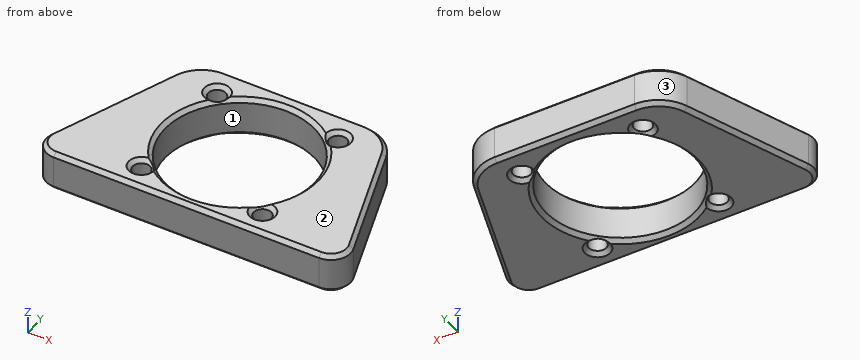
from build123d import *

# Parameters (mm, degrees)
SKETCH1_R           = 19
SKETCH1_R_2         = 2.25
BOSS_EXTRUDE1_DEPTH = 10
CHAMFER1_SIZE       = 1


with BuildPart() as part:
    # Sketch1 → Boss-Extrude1 (new body)
    with BuildSketch(Plane.XY):
        with BuildLine():
            Line((-27.380609914, 122.387194683), (-38.790304957, 90.693597341))
            ThreePointArc((-38.790304957, 90.693597341), (-38.176588293, 86.124933627), (-34.085867898, 84))
            Line((-34.085867898, 84), (-15.12911101, 84))
            Line((-15.12911101, 84), (15.12911101, 84))
            Line((15.12911101, 84), (34.085867898, 84))
            ThreePointArc((34.085867898, 84), (38.176588293, 86.124933627), (38.790304957, 90.693597341))
            Line((38.790304957, 90.693597341), (27.380609914, 122.387194683))
            ThreePointArc((27.380609914, 122.387194683), (23.721868541, 127.181440791), (17.971735796, 129))
            Line((17.971735796, 129), (-17.971735796, 129))
            ThreePointArc((-17.971735796, 129), (-23.721868541, 127.181440791), (-27.380609914, 122.387194683))
        make_face()
        with Locations(Location((0, 106, 0), (0, 0, 270))):
            Circle(SKETCH1_R, mode=Mode.SUBTRACT)
        with Locations(Location((15.556349182, 90.443650818, 0), (0, 0, 270))):
            Circle(SKETCH1_R_2, mode=Mode.SUBTRACT)
        with Locations(Location((-15.556349182, 90.443650818, 0), (0, 0, 270))):
            Circle(SKETCH1_R_2, mode=Mode.SUBTRACT)
        with Locations(Location((15.556349182, 121.556349182, 0), (0, 0, 270))):
            Circle(SKETCH1_R_2, mode=Mode.SUBTRACT)
        with Locations(Location((-15.556349182, 121.556349182, 0), (0, 0, 270))):
            Circle(SKETCH1_R_2, mode=Mode.SUBTRACT)
    extrude(amount=BOSS_EXTRUDE1_DEPTH)

    # Chamfer1
    # the kernel refuses this chamfer: 1 mm, written as the material it takes off along each edge
    with BuildSketch(Plane(origin=(17.971735796, 129, 0), x_dir=(0, 0.027495876610582174, 0.9996219169112968), z_dir=(-1, 0, 0)), Plane(origin=(17.971735796, 129, 10), x_dir=(0, -0.9996219169112968, 0.02749587661058574), z_dir=(-1, 0, 0))) as chamfer1_piece_1:
        Polygon((CHAMFER1_SIZE * 0.999621916911, -CHAMFER1_SIZE * 0.0274958766106), (-CHAMFER1_SIZE * 0.0274958766106, -CHAMFER1_SIZE * 0.999621916911), (0, 0), align=None)
    extrude(amount=35.943471591, mode=Mode.SUBTRACT)
    with BuildSketch(Plane(origin=(17.971735796, 119, 0), x_dir=(0.9408874118687268, 0.33871946827274174, 0), z_dir=(0.33871946827274174, -0.9408874118687268, 0))) as chamfer1_piece_2:
        Polygon((10, CHAMFER1_SIZE), (10 - CHAMFER1_SIZE, 0), (10, 0), align=None)
    revolve(axis=Axis((17.971735796, 119, 0), (0, 0, 1)), revolution_arc=70.201123645, mode=Mode.SUBTRACT)
    with BuildSketch(Plane(origin=(38.790304957, 90.693597341, 0), x_dir=(0.025870524181196484, 0.009313388705230746, 0.9996219169112968), z_dir=(-0.3387194682727421, 0.9408874118687267, 0)), Plane(origin=(-27.380609914, 122.387194683, 0), x_dir=(-0.025870524181196484, 0.00931338870523073, 0.9996219169112968), z_dir=(-0.3387194682727416, -0.9408874118687268, 0)), Plane(origin=(38.790304957, 90.693597341, 10), x_dir=(-0.9405316782499255, -0.33859140416997363, 0.027495876610585557), z_dir=(-0.3387194682727421, 0.9408874118687267, 0))) as chamfer1_piece_3:
        Polygon((CHAMFER1_SIZE * 0.999621916911, -CHAMFER1_SIZE * 0.0274958766106), (-CHAMFER1_SIZE * 0.0274958766106, -CHAMFER1_SIZE * 0.999621916911), (0, 0), align=None)
    extrude(amount=33.684792613, mode=Mode.SUBTRACT)
    with BuildSketch(Plane(origin=(34.085867898, 89, 0), x_dir=(0, -1, 0), z_dir=(-1, 0, 0))) as chamfer1_piece_4:
        Polygon((5, CHAMFER1_SIZE), (5 - CHAMFER1_SIZE, 0), (5, 0), align=None)
    revolve(axis=Axis((34.085867898, 89, 0), (0, 0, 1)), revolution_arc=109.798876355, mode=Mode.SUBTRACT)
    with BuildSketch(Plane(origin=(-34.085867898, 84, 0), x_dir=(0, -0.027495876610582174, 0.9996219169112968), z_dir=(1, 0, 0))) as chamfer1_piece_5:
        Polygon((CHAMFER1_SIZE * 0.999621916911, -CHAMFER1_SIZE * 0.0274958766106), (-CHAMFER1_SIZE * 0.0274958766106, -CHAMFER1_SIZE * 0.999621916911), (0, 0), align=None)
    extrude(amount=68.171735796, mode=Mode.SUBTRACT)
    with BuildSketch(Plane(origin=(-34.085867898, 89, 0), x_dir=(-0.9408874118687287, 0.33871946827273663, 0), z_dir=(0.33871946827273663, 0.9408874118687287, 0))) as chamfer1_piece_6:
        Polygon((5 - CHAMFER1_SIZE, 0), (5, CHAMFER1_SIZE), (5, 0), align=None)
    revolve(axis=Axis((-34.085867898, 89, 0), (0, 0, 1)), revolution_arc=109.798876355, mode=Mode.SUBTRACT)
    with BuildSketch(Plane(origin=(-17.971735796, 119, 0), x_dir=(0, 1, 0), z_dir=(1, 0, 0))) as chamfer1_piece_7:
        Polygon((10 - CHAMFER1_SIZE, 0), (10, CHAMFER1_SIZE), (10, 0), align=None)
    revolve(axis=Axis((-17.971735796, 119, 0), (0, 0, 1)), revolution_arc=70.201123645, mode=Mode.SUBTRACT)
    with BuildSketch(Plane(origin=(0, 106, 0), x_dir=(0, -1, 0), z_dir=(-1, 0, 0))) as chamfer1_piece_8:
        Polygon((19, CHAMFER1_SIZE), (19 + CHAMFER1_SIZE, 0), (19, 0), align=None)
    revolve(axis=Axis((0, 106, 0), (0, 0, 1)), mode=Mode.SUBTRACT)
    with BuildSketch(Plane(origin=(15.556349182, 90.443650818, 0), x_dir=(0, -1, 0), z_dir=(-1, 0, 0))) as chamfer1_piece_9:
        Polygon((2.25, CHAMFER1_SIZE), (2.25 + CHAMFER1_SIZE, 0), (2.25, 0), align=None)
    revolve(axis=Axis((15.556349182, 90.443650818, 0), (0, 0, 1)), mode=Mode.SUBTRACT)
    with BuildSketch(Plane(origin=(-15.556349182, 90.443650818, 0), x_dir=(0, -1, 0), z_dir=(-1, 0, 0))) as chamfer1_piece_10:
        Polygon((2.25, CHAMFER1_SIZE), (2.25 + CHAMFER1_SIZE, 0), (2.25, 0), align=None)
    revolve(axis=Axis((-15.556349182, 90.443650818, 0), (0, 0, 1)), mode=Mode.SUBTRACT)
    with BuildSketch(Plane(origin=(15.556349182, 121.556349182, 0), x_dir=(0, -1, 0), z_dir=(-1, 0, 0))) as chamfer1_piece_11:
        Polygon((2.25, CHAMFER1_SIZE), (2.25 + CHAMFER1_SIZE, 0), (2.25, 0), align=None)
    revolve(axis=Axis((15.556349182, 121.556349182, 0), (0, 0, 1)), mode=Mode.SUBTRACT)
    with BuildSketch(Plane(origin=(-15.556349182, 121.556349182, 0), x_dir=(0, -1, 0), z_dir=(-1, 0, 0))) as chamfer1_piece_12:
        Polygon((2.25, CHAMFER1_SIZE), (2.25 + CHAMFER1_SIZE, 0), (2.25, 0), align=None)
    revolve(axis=Axis((-15.556349182, 121.556349182, 0), (0, 0, 1)), mode=Mode.SUBTRACT)
    with BuildSketch(Plane(origin=(-17.971735796, 119, 10), x_dir=(0, 1, 0), z_dir=(1, 0, 0))) as chamfer1_piece_13:
        Polygon((10 - CHAMFER1_SIZE, 0), (10, -CHAMFER1_SIZE), (10, 0), align=None)
    revolve(axis=Axis((-17.971735796, 119, 10), (0, 0, 1)), revolution_arc=70.201123645, mode=Mode.SUBTRACT)
    with BuildSketch(Plane(origin=(-27.380609914, 122.387194683, 10), x_dir=(-0.025870524181196505, 0.009313388705230739, -0.9996219169112968), z_dir=(-0.3387194682727416, -0.9408874118687268, 0))) as chamfer1_piece_14:
        Polygon((CHAMFER1_SIZE * 0.999621916911, CHAMFER1_SIZE * 0.0274958766106), (-CHAMFER1_SIZE * 0.0274958766106, CHAMFER1_SIZE * 0.999621916911), (0, 0), align=None)
    extrude(amount=33.684792613, mode=Mode.SUBTRACT)
    with BuildSketch(Plane(origin=(-34.085867898, 89, 10), x_dir=(-0.9408874118687287, 0.33871946827273663, 0), z_dir=(0.33871946827273663, 0.9408874118687287, 0))) as chamfer1_piece_15:
        Polygon((5 - CHAMFER1_SIZE, 0), (5, -CHAMFER1_SIZE), (5, 0), align=None)
    revolve(axis=Axis((-34.085867898, 89, 10), (0, 0, 1)), revolution_arc=109.798876355, mode=Mode.SUBTRACT)
    with BuildSketch(Plane(origin=(34.085867898, 84, 10), x_dir=(0, 0.9996219169112968, 0.02749587661058574), z_dir=(-1, 0, 0))) as chamfer1_piece_16:
        Polygon((CHAMFER1_SIZE * 0.999621916911, CHAMFER1_SIZE * 0.0274958766106), (-CHAMFER1_SIZE * 0.0274958766106, CHAMFER1_SIZE * 0.999621916911), (0, 0), align=None)
    extrude(amount=68.171735796, mode=Mode.SUBTRACT)
    with BuildSketch(Plane(origin=(34.085867898, 89, 10), x_dir=(0, -1, 0), z_dir=(-1, 0, 0))) as chamfer1_piece_17:
        Polygon((5 - CHAMFER1_SIZE, 0), (5, -CHAMFER1_SIZE), (5, 0), align=None)
    revolve(axis=Axis((34.085867898, 89, 10), (0, 0, 1)), revolution_arc=109.798876355, mode=Mode.SUBTRACT)
    with BuildSketch(Plane(origin=(17.971735796, 119, 10), x_dir=(0.9408874118687268, 0.33871946827274174, 0), z_dir=(0.33871946827274174, -0.9408874118687268, 0))) as chamfer1_piece_18:
        Polygon((10 - CHAMFER1_SIZE, 0), (10, -CHAMFER1_SIZE), (10, 0), align=None)
    revolve(axis=Axis((17.971735796, 119, 10), (0, 0, 1)), revolution_arc=70.201123645, mode=Mode.SUBTRACT)
    with BuildSketch(Plane(origin=(0, 106, 10), x_dir=(0, -1, 0), z_dir=(-1, 0, 0))) as chamfer1_piece_19:
        Polygon((19 + CHAMFER1_SIZE, 0), (19, -CHAMFER1_SIZE), (19, 0), align=None)
    revolve(axis=Axis((0, 106, 10), (0, 0, 1)), mode=Mode.SUBTRACT)
    with BuildSketch(Plane(origin=(15.556349182, 90.443650818, 10), x_dir=(0, -1, 0), z_dir=(-1, 0, 0))) as chamfer1_piece_20:
        Polygon((2.25 + CHAMFER1_SIZE, 0), (2.25, -CHAMFER1_SIZE), (2.25, 0), align=None)
    revolve(axis=Axis((15.556349182, 90.443650818, 10), (0, 0, 1)), mode=Mode.SUBTRACT)
    with BuildSketch(Plane(origin=(-15.556349182, 90.443650818, 10), x_dir=(0, -1, 0), z_dir=(-1, 0, 0))) as chamfer1_piece_21:
        Polygon((2.25 + CHAMFER1_SIZE, 0), (2.25, -CHAMFER1_SIZE), (2.25, 0), align=None)
    revolve(axis=Axis((-15.556349182, 90.443650818, 10), (0, 0, 1)), mode=Mode.SUBTRACT)
    with BuildSketch(Plane(origin=(15.556349182, 121.556349182, 10), x_dir=(0, -1, 0), z_dir=(-1, 0, 0))) as chamfer1_piece_22:
        Polygon((2.25 + CHAMFER1_SIZE, 0), (2.25, -CHAMFER1_SIZE), (2.25, 0), align=None)
    revolve(axis=Axis((15.556349182, 121.556349182, 10), (0, 0, 1)), mode=Mode.SUBTRACT)
    with BuildSketch(Plane(origin=(-15.556349182, 121.556349182, 10), x_dir=(0, -1, 0), z_dir=(-1, 0, 0))) as chamfer1_piece_23:
        Polygon((2.25 + CHAMFER1_SIZE, 0), (2.25, -CHAMFER1_SIZE), (2.25, 0), align=None)
    revolve(axis=Axis((-15.556349182, 121.556349182, 10), (0, 0, 1)), mode=Mode.SUBTRACT)


solid = part.part
Check sheet for the modelled part. Datum: model origin and axes. Units: mm. Face numbers are marked on the shaded views. Give positions to 0.01 mm unless a question says otherwise; leave off trailing zeros. Write each loop counter-clockwise with the first axis right and the second up, starting at its lowest first coordinate (ties: lowest second). Pieces come first, ordered by that corner, then holes. Notation, with made-up numbers: (41, 21) -> (78, 21) arc R34 cw to (78, 54) -> close; hole circle Ø5 at (26.25, -22). An arc over 180 degrees is marked (long way). Write item = value, one per line.
Item 1: Sectioned sample at C-C on y = 106. Record the boundary of the cut face in (x, z).
Output:
outline = (-33.28, 1) -> (-32.22, 0) -> (-20, 0) -> (-19, 1) -> (-19, 9) -> (-20, 10) -> (-32.22, 10) -> (-33.28, 9) -> close; (19, 1) -> (20, 0) -> (32.22, 0) -> (33.28, 1) -> (33.28, 9) -> (32.22, 10) -> (20, 10) -> (19, 9) -> close
Item 2: Sectioned sample at B-B on z = 5.75. Record the boundary of the cut face in (x, y).
Output:
outline = (-38.79, 90.69) arc R5 ccw to (-34.09, 84) -> (34.09, 84) arc R5 ccw to (38.79, 90.69) -> (27.38, 122.39) arc R10 ccw to (17.97, 129) -> (-17.97, 129) arc R10 ccw to (-27.38, 122.39) -> close; hole circle Ø38 at (0, 106); hole circle Ø4.5 at (-15.56, 90.44); hole circle Ø4.5 at (-15.56, 121.56); hole circle Ø4.5 at (15.56, 90.44); hole circle Ø4.5 at (15.56, 121.56)
Item 3: Release check for a two-part mould opening along X. For the marked faces 1, 2 and 3 record: +X half, -X half, draft (parallel to the pull), parting line (faces both ways), or undercut.
Output:
face_1 = undercut
face_2 = draft
face_3 = -X half
Item 4: Scan lines: probe 1 along X at (y, z) = (123, 1.5); probe 2 along X at (y, z) = (106, 3); probe 3 along X at (y, z) = (99, 4). Record each from-to range of solid material in increasing order. Write a range as from..to.
Output:
probe_1 = -27.14..-17.28, -13.83..-8.49, 8.49..13.83, 17.28..27.14
probe_2 = -33.28..-19, 19..33.28
probe_3 = -35.8..-17.66, 17.66..35.8
Item 5: Gauge pin test, flat ends, axial feed: pin 1 (4 mm diameter, centred on x = 15.56, y = 90.44, fed in from -Z); pin 2 (5 mm diameter, centred on x = -15.56, y = 90.44, fed in from +Z); pin 3 (1 mm diameter, centred on y = 107.5, z = 4.5, fed in from +X); pin 4 (6 mm diameter, centred on x = 15.56, y = 121.56, fed in from -Z). Record the tip position at first contact, or that the pin passes through.
Output:
pin_1 = through
pin_2 = 9.26
pin_3 = 32.92
pin_4 = 0.24
Item 6: Sectioned sample at A-A on x = 0. Record the boundary of the cut face in (y, z).
Output:
outline = (84, 1) -> (85, 0) -> (86, 0) -> (87, 1) -> (87, 9) -> (86, 10) -> (85, 10) -> (84, 9) -> close; (125, 1) -> (126, 0) -> (128, 0) -> (129, 1) -> (129, 9) -> (128, 10) -> (126, 10) -> (125, 9) -> close
